from build123d import *

# Parameters (mm, degrees)
SKETCH_1_W          = 50
SKETCH_1_H          = 50
SKETCH_1_R          = 14
SKETCH_1_R_2        = 2.5
EXTRUDE_1_DEPTH     = 2
SKETCH_3_W          = 2
SKETCH_3_H          = 50
EXTRUDE_3_DEPTH     = 48
EXTRUDE_4_DEPTH     = 2
EXTRUDE_5_DEPTH     = 2
SKETCH_6_R          = 13
SKETCH_6_R_2        = 2
CUT_EXTRUDE_1_DEPTH = 2
FILLET_1_R          = 5


with BuildPart() as part:
    # 草图1 → 凸台-拉伸1 (new body)
    with BuildSketch(Plane.XY):
        Rectangle(SKETCH_1_W, SKETCH_1_H)
        with Locations((-1, 0)):
            Circle(SKETCH_1_R, mode=Mode.SUBTRACT)
        with Locations((-16, 15)):
            Circle(SKETCH_1_R_2, mode=Mode.SUBTRACT)
        with Locations(Location((-16, -15, 0), (0, 0, 180))):
            Circle(SKETCH_1_R_2, mode=Mode.SUBTRACT)
        with Locations((14, -15)):
            Circle(SKETCH_1_R_2, mode=Mode.SUBTRACT)
        with Locations(Location((14, 15, 0), (0, 0, 180))):
            Circle(SKETCH_1_R_2, mode=Mode.SUBTRACT)
    extrude(amount=EXTRUDE_1_DEPTH)

    # 草图3 → 凸台-拉伸3 (add)
    with BuildSketch(Plane(origin=(0, 0, 0), x_dir=(-1, 0, 0), z_dir=(0, 0, -1))):
        with Locations((-24, 0)):
            Rectangle(SKETCH_3_W, SKETCH_3_H)
    extrude(amount=EXTRUDE_3_DEPTH)

    # 草图4 → 凸台-拉伸4 (add)
    with BuildSketch(Plane(origin=(0, 25, 0), x_dir=(1, 0, 0), z_dir=(0, 1, 0))):
        Polygon((0, -2), (25, 23), (25, -2), align=None)
    extrude(amount=-EXTRUDE_4_DEPTH)

    # 草图5 → 凸台-拉伸5 (add)
    with BuildSketch(Plane.XZ.offset(25)):
        Polygon((25, 2), (0, 2), (25, -23), align=None)
    extrude(amount=-EXTRUDE_5_DEPTH)

    # 草图6 → 切除-拉伸1 (cut)
    with BuildSketch(Plane(origin=(25, 0, 0), x_dir=(0, 0, -1), z_dir=(1, 0, 0))):
        with Locations(Location((26, 0, 0), (0, 0, 90))):
            Circle(SKETCH_6_R)
        with Locations(Location((43.5, 0, 0), (0, 0, 90))):
            Circle(SKETCH_6_R_2)
        with Locations(Location((26, 17.5, 0), (0, 0, 90))):
            Circle(SKETCH_6_R_2)
        with Locations(Location((26, -17.5, 0), (0, 0, 270))):
            Circle(SKETCH_6_R_2)
        with Locations(Location((8.5, 0, 0), (0, 0, 270))):
            Circle(SKETCH_6_R_2)
    extrude(amount=-CUT_EXTRUDE_1_DEPTH, mode=Mode.SUBTRACT)

    # 圆角1
    fillet_1_edges = [part.edges().sort_by_distance(p)[0] for p in [
        (24, -25, -48),
        (24, 25, -48),
        (-25, -25, 1),
        (-25, 25, 1),
    ]]
    fillet(fillet_1_edges, radius=FILLET_1_R)


solid = part.part
Can you work these out from the model? Positions are in its coordinate system, mm. A direction names the side the tool comes from. Coordinates: 2 decimals unless noted, no trailing zeros. Write each loop counter-clockwise with the first axis right and the second up, starting at its lowest first coordinate (ties: lowest second). Pieces come first, ordered by that corner, then holes. Notation, with made-up numbers: (86, 59.5) - (138, 59.5) arc R22 ccw to (138, 93.5) - close; hole circle Ø5 at (-8, 41.5). An arc over 180 degrees is marked (long way). Return JSON: item names as keys, results as strings. Group by question number.
Item 1: Please list where these lines run through material, in increasing order: probe 1 along Z at (x, y) = (24, 0); probe 2 along Z at (x, y) = (23.65, 17.5); probe 3 along Y at (x, z) = (-1, 1.3).
Item 2: If we section it at B-B (x = -16): Write out the boundary of the cut face in (y, z), then the cut area to 3 significant figures.
Item 3: Which directions (+Z, -Z, +X, -X, +Y, -Y) give clear straight access to the entire face, cutting with the end or side of a thin tool? Please do faces 5 (the face through (24, -24, -46)), 6 (the face through (23, -6, -13)).
Item 4: I'm going to push flat-ended pins straight in: pin 1 Ø3 at (y, z) = (11, -11.5) entering from -X; pin 2 Ø5 at (y, z) = (-17.5, -26) entering from +X; pin 3 Ø2.5 at (y, z) = (17.5, -26) entering from -X; pin 4 Ø24 at (x, y) = (-3, 11.5) entering from -Z. Where does each tip first touch, or does it pass through?
Item 5: If we section it at D-D (y = -5.5): Write out the boundary of the cut face in (x, z).
Item 6: If we section it at C-C (z = -2.5): Write out the boundary of the cut face in (x, y), then the cut area to 3 significant figures.
Item 7: We'd pull the mould along X, two halves only. Please class faces 1 (the face through (25, 0, -12)), 2 (the face through (11.5, -14.9, 1)), 3 (the face through (24.01, -9.58, -17.21)), 4 (the face through (-13.5, -15.1, 1)): pulls with the +X half, pulls with the -X half, needs draft (parallel to the pull), parting line crosses it, or undercut.
Item 8: If we section it at A-A (z = -26): Write out the boundary of the cut face in (x, y).
Return value:
{
 "1": {"probe 1": "z = -48 to -45.5, -41.5 to -39, -13 to -10.5, -6.5 to 2", "probe 2": "z = -48 to -28, -24 to 2", "probe 3": "y = -25 to -14, 14 to 25"},
 "2": {"outline": "(-25, 0) - (-17.5, 0) - (-17.5, 2) - (-25, 2) - close; (-12.5, 0) - (12.5, 0) - (12.5, 2) - (-12.5, 2) - close; (17.5, 0) - (25, 0) - (25, 2) - (17.5, 2) - close", "area": "80.0 mm^2"},
 "3": {"face 5": "-Z, +X, -X, -Y", "face 6": "-Z, -X"},
 "4": {"pin 1": "stops at x = 23", "pin 2": "stops at x = 25", "pin 3": "passes through", "pin 4": "stops at z = 0"},
 "5": {"outline": "(-25, 0) - (-13.87, 0) - (-13.87, 2) - (-25, 2) - close; (11.87, 0) - (23, 0) - (23, -14.22) - (25, -14.22) - (25, 2) - (11.87, 2) - close; (23, -48) - (25, -48) - (25, -37.78) - (23, -37.78) - close"},
 "6": {"outline": "(4.5, -25) - (25, -25) - (25, 25) - (4.5, 25) - (4.5, 23) - (23, 23) - (23, -23) - (4.5, -23) - close", "area": "174 mm^2"},
 "7": {"face 1": "pulls with the +X half", "face 2": "undercut", "face 3": "needs draft", "face 4": "undercut"},
 "8": {"outline": "(23, -25) - (25, -25) - (25, -19.5) - (23, -19.5) - close; (23, -15.5) - (25, -15.5) - (25, -13) - (23, -13) - close; (23, 13) - (25, 13) - (25, 15.5) - (23, 15.5) - close; (23, 19.5) - (25, 19.5) - (25, 25) - (23, 25) - close"}
}
